The model under review builds one solid part; all positions refer to its coordinate system, in mm. Round coordinates to 2 decimals unless told otherwise and drop trailing zeros.
Item 1: Clearance check with flat-ended pins moving along their axes: pin 1 Ø3.5 at (x, y) = (0, 0) entering from +Z; pin 2 Ø2.5 at (x, y) = (0, 0) entering from +Z. State where each tip first meets the part, or that it passes through.
Item 2: To check wall thickness, follow L1, parallel to Y at x = 0, z = -1.2; L2, parallel to Y at x = -1, z = -1.1; L3, parallel to X at y = 0.5, z = -1.4. State the ranges of each line that lie inside material, in increasing order.
Item 3: Add section A-A (x = 1.75). State how many separate pieces and enclosed holes the cut face has, plus the area to 3 significant figures.
```python
from build123d import *

# Parameters (mm, degrees)
SKETCH5_W               = 2.2
SKETCH5_H               = 7
SKETCH7_W               = 2.2
SKETCH7_H               = 2
SKETCH9_W               = 2.2
SKETCH9_H               = 0.454663337
THREAD_SIMPLE_COUNT     = 4
THREAD_SIMPLE_PITCH     = 0.7
SKETCH22_OUTSIDE_W      = 15.9
SKETCH22_OUTSIDE_H      = 15.9
CUT_PROFILE_OUTER_DEPTH = 3.2


with BuildPart() as part:
    # Sketch5 → body (revolve)
    with BuildSketch(Plane(origin=(0, 0, 0), x_dir=(0, 0, -1), z_dir=(1, 0, 0))):
        with Locations((1.1, 3.5)):
            Rectangle(SKETCH5_W, SKETCH5_H)
    revolve(axis=Axis((0, 0, 0), (0, 0, -1)))

    # Sketch19 → cut-chamfer-start (revolve, cut)
    with BuildSketch(Plane(origin=(0, 0, 0), x_dir=(0, 0, -1), z_dir=(1, 0, 0))):
        Polygon((2.020725942, -7), (0, -7), (0, -3.5), align=None)
    revolve(axis=Axis((0, 0, 0), (0, 0, -1)), mode=Mode.SUBTRACT)

    # Sketch20 → cut-chamfer-end (revolve, cut)
    with BuildSketch(Plane(origin=(0, 0, 0), x_dir=(0, 0, -1), z_dir=(1, 0, 0))):
        Polygon((2.2, -7), (0.179274058, -7), (2.2, -3.5), align=None)
    revolve(axis=Axis((0, 0, 0), (0, 0, -1)), mode=Mode.SUBTRACT)

    # Sketch7 → body-bore (revolve, cut)
    with BuildSketch(Plane(origin=(0, 0, 0), x_dir=(0, 0, -1), z_dir=(1, 0, 0))):
        with Locations((1.1, 1)):
            Rectangle(SKETCH7_W, SKETCH7_H)
    revolve(axis=Axis((0, 0, -2.2), (0, 0, 1)), mode=Mode.SUBTRACT)

    # Sketch9 → body-thread (revolve)
    with BuildSketch(Plane(origin=(0, 0, 0), x_dir=(0, 0, -1), z_dir=(1, 0, 0))):
        with Locations((1.1, -1.848445555)):
            Rectangle(SKETCH9_W, SKETCH9_H)
    revolve(axis=Axis((0, 0, 0), (0, 0, -1)))

    # Sketch10 → thread-single (revolve, cut)
    with BuildSketch(Plane(origin=(0, 0, 0), x_dir=(0, 0, -1), z_dir=(1, 0, 0))):
        with BuildLine():
            Line((2.15625, -2), (1.9375, -1.621113886))
            Line((1.9375, -1.621113886), (2.4625, -1.621113886))
            Line((2.4625, -1.621113886), (2.24375, -2))
            ThreePointArc((2.24375, -2), (2.2, -2.025259074), (2.15625, -2))
        make_face()
    thread_single = revolve(axis=Axis((0, 0, 0), (0, 0, -1)), mode=Mode.SUBTRACT)

    # thread-simple: thread-single ×4
    with Locations(*[(0, 0, i * THREAD_SIMPLE_PITCH) for i in range(1, THREAD_SIMPLE_COUNT)]):
        add(thread_single, mode=Mode.SUBTRACT)

    # Sketch15 → cut-chamfer-start-inner (revolve, cut)
    with BuildSketch(Plane(origin=(0, 0, 0), x_dir=(0, 0, -1), z_dir=(1, 0, 0))):
        Polygon((0, -1.621113886), (0.454663337, -1.621113886), (0, -2.075777223), align=None)
    revolve(axis=Axis((0, 0, 0), (0, 0, -1)), mode=Mode.SUBTRACT)

    # Sketch16 → cut-chamfer-end-inner (revolve, cut)
    with BuildSketch(Plane(origin=(0, 0, 0), x_dir=(0, 0, -1), z_dir=(1, 0, 0))):
        Polygon((2.2, -1.621113886), (2.2, -2.075777223), (1.745336663, -1.621113886), align=None)
    revolve(axis=Axis((0, 0, 0), (0, 0, -1)), mode=Mode.SUBTRACT)

    # Sketch22 outside → cut-profile-outer (cut, through all)
    with BuildSketch(Plane.XY):
        Rectangle(SKETCH22_OUTSIDE_W, SKETCH22_OUTSIDE_H)
        Polygon((4.041451884, 0), (2.020725942, 3.5), (-2.020725942, 3.5), (-4.041451884, 0), (-2.020725942, -3.5), (2.020725942, -3.5), align=None, mode=Mode.SUBTRACT)
    extrude(amount=-CUT_PROFILE_OUTER_DEPTH, mode=Mode.SUBTRACT)


solid = part.part
```
Numbers:
1. pin 1: stops at z = -0.33
1. pin 2: passes through
2. L1: y = -3.5 to -1.62, 1.62 to 3.5
2. L2: y = -3.5 to -1.28, 1.28 to 3.5
2. L3: x = -3.75 to -1.84, 1.84 to 3.75
3. separate pieces: 1
3. enclosed holes: 2
3. area: 13.1 mm2
